from build123d import *

# Parameters (mm, degrees)
SKETCH2_R           = 10
BOSS_EXTRUDE1_DEPTH = 2
SKETCH2_3_R         = 4.5
SKETCH2_3_R_2       = 2.75
BOSS_EXTRUDE2_DEPTH = 4.5
CIRPATTERN1_COUNT   = 4


with BuildPart() as part:
    # Sketch2 → Boss-Extrude1 (new body)
    with BuildSketch(Plane(origin=(0, 0, 0), x_dir=(1, 0, 0), z_dir=(0, 1, 0))):
        with Locations(Location((0, 0, 0), (0, 0, 270))):
            Circle(SKETCH2_R)
    extrude(amount=-BOSS_EXTRUDE1_DEPTH)

    # Sketch2_3 → Boss-Extrude2 (add)
    with BuildSketch(Plane(origin=(0, 0, 0), x_dir=(1, 0, 0), z_dir=(0, 1, 0))):
        with Locations(Location((0, 0, 0), (0, 0, 270))):
            Circle(SKETCH2_3_R)
        with Locations(Location((0, 0, 0), (0, 0, 270))):
            Circle(SKETCH2_3_R_2, mode=Mode.SUBTRACT)
    extrude(amount=BOSS_EXTRUDE2_DEPTH)

    # Sketch5 → Tap Drill for M3x0.5 Tap1 (revolve, cut)
    with BuildSketch(Plane(origin=(0, 0, -7), x_dir=(0, 0, 1), z_dir=(1, 0, 0))):
        Polygon((0, 0), (0, 10.911075774), (1.25, 10.16), (1.25, 0), align=None)
    tap_drill_for_m3x0_5_tap1 = revolve(axis=Axis((0, 6.35, -7), (0, -1, 0)), mode=Mode.SUBTRACT)

    # CirPattern1: Tap Drill for M3x0.5 Tap1 ×4 about axis
    cirpattern1_axis = Axis((0, 0, 0), (0, 1, 0))
    for i in range(1, CIRPATTERN1_COUNT):
        add(tap_drill_for_m3x0_5_tap1.rotate(cirpattern1_axis, i * 360 / CIRPATTERN1_COUNT), mode=Mode.SUBTRACT)


solid = part.part
Part model, mm, in its own coordinate system. A direction names the side the tool comes from. Give positions to 0.01 mm unless a question says otherwise; leave off trailing zeros. Loops run counter-clockwise (first coordinate to the right, second up) from the corner with the lowest first, then second, coordinate; pieces in that order, holes last.
(1) Pin check, flat tips, straight feed: pin 1 (1 mm diameter, centred on x = -4, y = 2, fed in from +Z); pin 2 (1 mm diameter, centred on x = -4, y = 2, fed in from -Z); pin 3 (1 mm diameter, centred on y = -0.5, z = -2.5, fed in from +X). Stop position of each tip, or through.
Return value:
pin 1: stops at z = 2.83
pin 2: stops at z = -2.83
pin 3: stops at x = 9.8
(2) Band-saw the part on D-D (y = -0.25). Write the cut outline in (x, z).
Return value:
outline: circle Ø20 at (0, 0); hole circle Ø2.5 at (-7, 0); hole circle Ø2.5 at (0, -7); hole circle Ø2.5 at (0, 7); hole circle Ø2.5 at (7, 0)
(3) Pull direction Z, two halves, no side cores. Call faces 1 (the flat face through (-3, 4.5, 0)), 2 (the cylindrical face through (-2.685, 2.218, -0.596)), 3 (the cylindrical face through (1.352, 2.218, 4.292)), 4 (the cylindrical face through (-8.25, -0.99, 0.05)): pulls with the +Z half, pulls with the -Z half, needs draft (parallel to the pull), parting line crosses it, or undercut.
Return value:
face 1: needs draft
face 2: undercut
face 3: parting line crosses it
face 4: undercut
(4) Band-saw the part on C-C (x = 0). Write the cut outline in (y, z).
Return value:
outline: (-2, -10) - (0, -10) - (0, -8.25) - (-2, -8.25) - close; (-2, -5.75) - (0, -5.75) - (0, -4.5) - (4.5, -4.5) - (4.5, -2.75) - (0, -2.75) - (0, 2.75) - (4.5, 2.75) - (4.5, 4.5) - (0, 4.5) - (0, 5.75) - (-2, 5.75) - close; (-2, 8.25) - (0, 8.25) - (0, 10) - (-2, 10) - close
(5) Band-saw the part on B-B (z = 0). Write the cut outline in (x, y).
Return value:
outline: (-10, -2) - (-8.25, -2) - (-8.25, 0) - (-10, 0) - close; (-5.75, -2) - (5.75, -2) - (5.75, 0) - (4.5, 0) - (4.5, 4.5) - (2.75, 4.5) - (2.75, 0) - (-2.75, 0) - (-2.75, 4.5) - (-4.5, 4.5) - (-4.5, 0) - (-5.75, 0) - close; (8.25, -2) - (10, -2) - (10, 0) - (8.25, 0) - close
(6) Drill centre lines: line 1 along Z through (x, y) = (-0.75, -0.5); line 2 along X through (y, z) = (2.25, 0); line 3 along Y through (x, z) = (-0.75, -2.25). Where is each one in solid material? Low to high.
Return value:
line 1: z = -9.97 to -8, -6 to 6, 8 to 9.97
line 2: x = -4.5 to -2.75, 2.75 to 4.5
line 3: y = -2 to 0
(7) Band-saw the part on A-A (x = 7). Write the cut outline in (y, z), and give its area (3 significant figures).
Return value:
outline: (-2, -7.14) - (0, -7.14) - (0, -1.25) - (-2, -1.25) - close; (-2, 1.25) - (0, 1.25) - (0, 7.14) - (-2, 7.14) - close
area: 23.6 mm2
(8) 3-axis set-ups, long thin cutter, end or side, ignore diameter. For faces 5 (the flat face through (0, 0, 0)), 6 (the cylindrical face through (8.25, -0.99, -0.05)): which of +Z, -Z, +X, -X, +Y, -Y reach the whole face in a straight line?
Return value:
face 5: +Y
face 6: +Y, -Y
